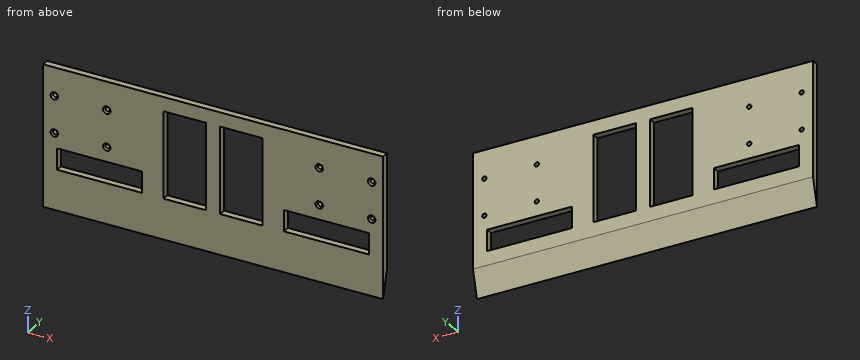
from build123d import *

# Parameters (mm, degrees)
SKETCH_1_W          = 240
SKETCH_1_H          = 100
EXTRUDE_1_DEPTH     = 2.5
CUT_EXTRUDE_1_DEPTH = 261.012018953
SKETCH_3_R          = 1.5
CUT_EXTRUDE_2_DEPTH = 261.048072479
SKETCH_5_W          = 70
SKETCH_5_H          = 61.339745962
CUT_EXTRUDE_4_DEPTH = 10
SKETCH_6_W          = 60
SKETCH_6_H          = 15
CUT_EXTRUDE_5_DEPTH = 10
SKETCH_7_W          = 10
SKETCH_7_H          = 5
EXTRUDE_2_DEPTH     = 70
CHAMFER_1_SIZE      = 1.12


with BuildPart() as part:
    # 草图1 → 凸台-拉伸1 (new, symmetric)
    with BuildSketch(Plane(origin=(0, 0, 0), x_dir=(1, 0, 0), z_dir=(0, 1, 0))):
        with Locations((120, -50)):
            Rectangle(SKETCH_1_W, SKETCH_1_H)
    extrude(amount=EXTRUDE_1_DEPTH, both=True)

    # 草图2 → 切除-拉伸1 (cut, through all)
    with BuildSketch(Plane(origin=(240, 0, 0), x_dir=(0, 0, -1), z_dir=(1, 0, 0))):
        Polygon((0, -2.5), (-18.660254038, 2.5), (0, 2.5), align=None)
    extrude(amount=-CUT_EXTRUDE_1_DEPTH, mode=Mode.SUBTRACT)

    # 草图3 → 切除-拉伸2 (cut, through all)
    with BuildSketch(Plane(origin=(0, 2.5, 0), x_dir=(1, 0, 0), z_dir=(0, 1, 0))):
        with Locations(Location((45, -80, 0), (0, 0, 270))):
            Circle(SKETCH_3_R)
        with Locations(Location((45, -54, 0), (0, 0, 90))):
            Circle(SKETCH_3_R)
        with Locations(Location((8, -80, 0), (0, 0, 90))):
            Circle(SKETCH_3_R)
        with Locations(Location((8, -54, 0), (0, 0, 270))):
            Circle(SKETCH_3_R)
        with Locations(Location((195, -80, 0), (0, 0, 90))):
            Circle(SKETCH_3_R)
        with Locations(Location((195, -54, 0), (0, 0, 270))):
            Circle(SKETCH_3_R)
        with Locations(Location((232, -80, 0), (0, 0, 270))):
            Circle(SKETCH_3_R)
        with Locations(Location((232, -54, 0), (0, 0, 90))):
            Circle(SKETCH_3_R)
    extrude(amount=-CUT_EXTRUDE_2_DEPTH, mode=Mode.SUBTRACT)

    # 草图5 → 切除-拉伸4 (cut)
    with BuildSketch(Plane(origin=(0, 2.5, 0), x_dir=(1, 0, 0), z_dir=(0, 1, 0))):
        with Locations((120, -59.330127019)):
            Rectangle(SKETCH_5_W, SKETCH_5_H)
    extrude(amount=-CUT_EXTRUDE_4_DEPTH, mode=Mode.SUBTRACT)

    # 草图6 → 切除-拉伸5 (cut)
    with BuildSketch(Plane(origin=(0, 2.5, 0), x_dir=(1, 0, 0), z_dir=(0, 1, 0))):
        with Locations((40, -36.160254038)):
            Rectangle(SKETCH_6_W, SKETCH_6_H)
        with Locations((200, -36.160254038)):
            Rectangle(SKETCH_6_W, SKETCH_6_H)
    extrude(amount=-CUT_EXTRUDE_5_DEPTH, mode=Mode.SUBTRACT)

    # 草图7 → 凸台-拉伸2 (add)
    with BuildSketch(Plane.XY.offset(28.660254038)):
        with Locations((120, 0)):
            Rectangle(SKETCH_7_W, SKETCH_7_H)
    extrude(amount=EXTRUDE_2_DEPTH)

    # 倒角1
    chamfer_1_edges = [part.edges().sort_by_distance(p)[0] for p in [
        (195, -2.5, 81.5),
        (8, -2.5, 52.5),
        (8, -2.5, 81.5),
        (45, -2.5, 55.5),
        (232, -2.5, 55.5),
        (232, -2.5, 78.5),
        (195, -2.5, 52.5),
        (45, -2.5, 78.5),
    ]]
    chamfer(chamfer_1_edges, length=CHAMFER_1_SIZE)


solid = part.part
Geometry check sheet. Reference: the model listing, model coordinates, mm. Round coordinates to 2 decimals unless told otherwise and drop trailing zeros. Write each loop counter-clockwise with the first axis right and the second up, starting at its lowest first coordinate (ties: lowest second). Pieces come first, ordered by that corner, then holes. Notation, with made-up numbers: (77.25, 61) - (100.25, 61) arc R11 ccw to (100.25, 78) - close; hole circle Ø1 at (42.25, 25.25). An arc over 180 degrees is marked (long way). One line per item, written item: value.
1. Cross-section at C-C on z = 72. Record the boundary of the cut face in (x, y).
The answers:
outline: (0, -2.5) - (85, -2.5) - (85, 2.5) - (0, 2.5) - close; (115, -2.5) - (125, -2.5) - (125, 2.5) - (115, 2.5) - close; (155, -2.5) - (240, -2.5) - (240, 2.5) - (155, 2.5) - close
2. Cross-section at D-D on y = -0.05. Give the number of separate pieces and of enclosed holes in the cut face, and give its area (3 significant figures).
The answers:
separate pieces: 1
enclosed holes: 12
area: 16,300 mm^2
3. Cross-section at B-B on x = 203. Record the boundary of the cut face in (y, z), and give its area (3 significant figures).
The answers:
outline: (-2.5, 0) - (2.5, 18.66) - (2.5, 28.66) - (-2.5, 28.66) - close; (-2.5, 43.66) - (2.5, 43.66) - (2.5, 100) - (-2.5, 100) - close
area: 378 mm^2
4. Cross-section at A-A on z = 35. Record the boundary of the cut face in (x, y).
The answers:
outline: (0, -2.5) - (10, -2.5) - (10, 2.5) - (0, 2.5) - close; (70, -2.5) - (85, -2.5) - (85, 2.5) - (70, 2.5) - close; (115, -2.5) - (125, -2.5) - (125, 2.5) - (115, 2.5) - close; (155, -2.5) - (170, -2.5) - (170, 2.5) - (155, 2.5) - close; (230, -2.5) - (240, -2.5) - (240, 2.5) - (230, 2.5) - close
5. Scan lines: L1, parallel to X at y = -1.35, z = 43; L2, parallel to X at y = 1.9, z = 44; L3, parallel to Y at x = 71, z = 9.5. Record each from-to range of solid material in increasing order.
The answers:
L1: x = 0 to 10, 70 to 85, 115 to 125, 155 to 170, 230 to 240
L2: x = 0 to 85, 115 to 125, 155 to 240
L3: y = -2.5 to 0.05
